Job drawing, mm, ordinate dimensions from the low corner. One solid piece. A direction names the side the tool comes from. Give positions to 0.01 mm unless a question says otherwise; leave off trailing zeros. Loops run counter-clockwise (first coordinate to the right, second up) from the corner with the lowest first, then second, coordinate; pieces in that order, holes last. Notation, with made-up numbers: (9, 49.25) - (29, 49.25) arc R13 ccw to (29, 67.25) - close; hole circle Ø1 at (2.5, 80). An arc over 180 degrees is marked (long way). Use a Markdown table: item, result.
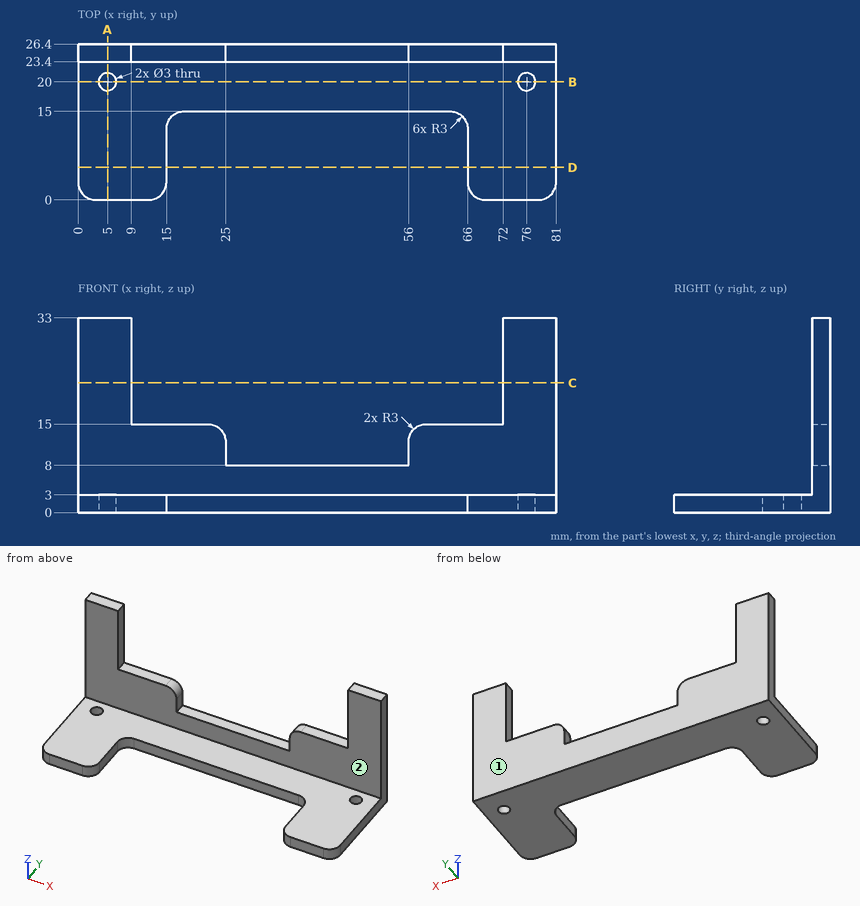
(1) Slice it at B-B, the plane y = 20. Write the cut outline in (x, z), plus the area to 3 significant figures.
Computed:
| item | result |
|---|---|
| outline | (0, 0) - (3.5, 0) - (3.5, 3) - (0, 3) - close; (6.5, 0) - (74.5, 0) - (74.5, 3) - (6.5, 3) - close; (77.5, 0) - (81, 0) - (81, 3) - (77.5, 3) - close |
| area | 225 mm² |
(2) Slice it at A-A, the plane x = 5. Write the cut outline in (y, z).
Computed:
| item | result |
|---|---|
| outline | (0, 0) - (18.5, 0) - (18.5, 3) - (0, 3) - close; (21.5, 0) - (26.4, 0) - (26.4, 33) - (23.4, 33) - (23.4, 3) - (21.5, 3) - close |
(3) Slice it at C-C, the plane z = 22. Write the cut outline in (x, y).
Computed:
| item | result |
|---|---|
| outline | (0, 23.4) - (9, 23.4) - (9, 26.4) - (0, 26.4) - close; (72, 23.4) - (81, 23.4) - (81, 26.4) - (72, 26.4) - close |
(4) Pin check, flat tips, straight feed: P1, Ø3.5, axis at x = 5, y = 20, coming from the +Z side; P2, Ø3.5, axis at x = 35, y = 25.5, coming from the +Z side; P3, Ø0.9, axis at x = 29.5, z = 1, coming from the -Y side. Stop position of each tip, or through.
Computed:
| item | result |
|---|---|
| P1 | z = 3 |
| P2 | z = 8 |
| P3 | y = 15 |
(5) Drill centre lines: probe 1 along Y at (x, z) = (5, 1.85); probe 2 along Z at (x, y) = (74, 6.75); probe 3 along Y at (x, z) = (9, 8.5). Where is each one in solid material? Low to high. Write a range as [from, to].
Computed:
| item | result |
|---|---|
| probe 1 | [0, 18.5], [21.5, 26.4] |
| probe 2 | [0, 3] |
| probe 3 | [23.4, 26.4] |
(6) Slice it at D-D, the plane y = 5.5. Write the cut outline in (x, z), plus the area to 3 significant figures.
Computed:
| item | result |
|---|---|
| outline | (0, 0) - (15, 0) - (15, 3) - (0, 3) - close; (66, 0) - (81, 0) - (81, 3) - (66, 3) - close |
| area | 90.0 mm² |
(7) 3-axis set-ups, long thin cutter, end or side, ignore diameter. For the marked faces 1 and 2: which of +Z, -Z, +X, -X, +Y, -Y reach the whole face in a straight line?
Computed:
| item | result |
|---|---|
| face 1 | +Z, -Z, +X, -X, +Y |
| face 2 | +Z, +X, -X, -Y |
